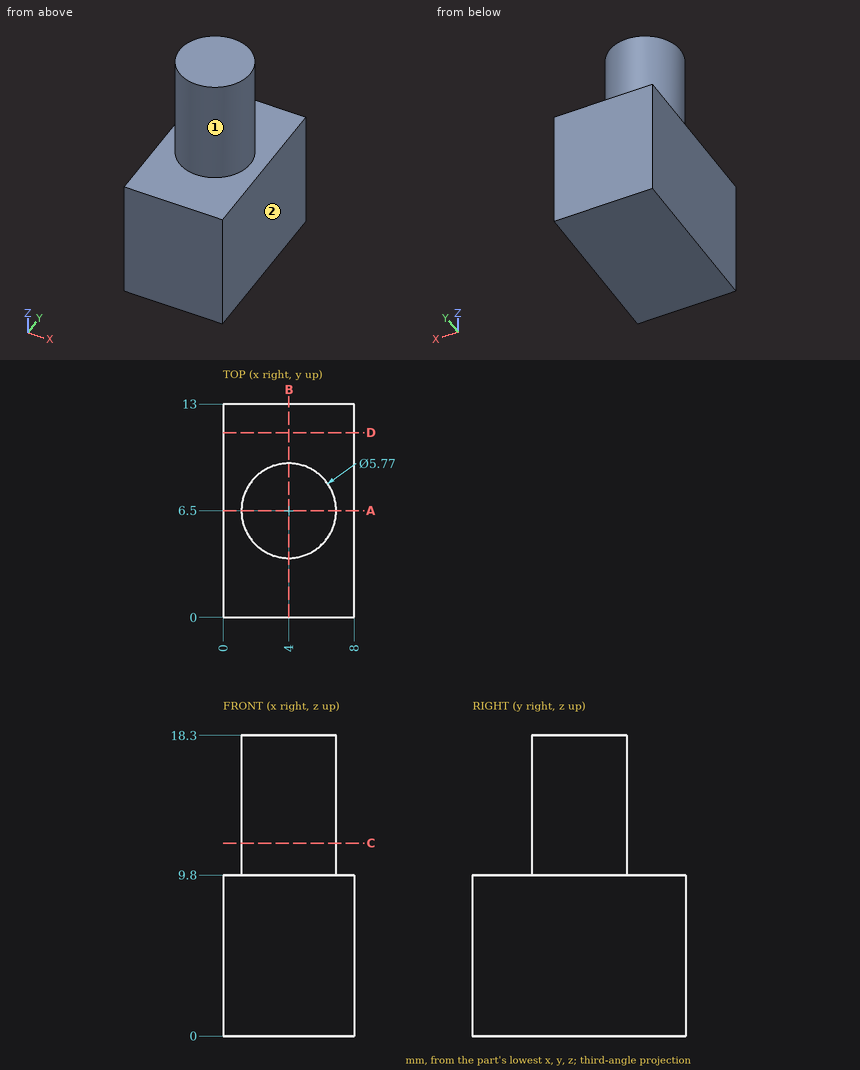
Print and shaded views of the part. All mm, measured from the part's lowest x, y and z. A direction names the side the tool comes from. Give positions to 0.01 mm unless a question says otherwise; leave off trailing zeros. Loops run counter-clockwise (first coordinate to the right, second up) from the corner with the lowest first, then second, coordinate; pieces in that order, holes last. Notation, with made-up numbers: (-31.75, -4.5) -> (25.25, -4.5) arc R22 ccw to (25.25, 11.5) -> close; hole circle Ø11 at (-18.75, 20). An arc over 180 degrees is marked (long way). Answer in a Markdown table with one row per item.
Item 1: Slice it at D-D on y = 11.25. Write the cut outline in (x, z), plus the area to 3 significant figures.
Findings below:
| item | result |
|---|---|
| outline | (0, 0) -> (8, 0) -> (8, 9.8) -> (0, 9.8) -> close |
| area | 78.4 mm² |
Item 2: Slice it at A-A on y = 6.5. Write the cut outline in (x, z) (3 decimals), plus the area to 3 significant figures.
Findings below:
| item | result |
|---|---|
| outline | (0, 0) -> (8, 0) -> (8, 9.8) -> (6.885, 9.8) -> (6.885, 18.3) -> (1.115, 18.3) -> (1.115, 9.8) -> (0, 9.8) -> close |
| area | 127 mm² |
Item 3: Tool access for the marked faces 1 and 2: list every direction of +Z, -Z, +X, -X, +Y, -Y with a clear straight run to the whole face (end or side of a thin tool).
Findings below:
| item | result |
|---|---|
| face 1 | +Z |
| face 2 | +Z, -Z, +X, +Y, -Y |
Item 4: Flat gauge pins, fed straight in: P1, Ø3, axis at y = 9, z = 5.5, coming from the -X side; P2, Ø3, axis at x = 2, z = 15.5, coming from the -Y side; P3, Ø1, axis at x = 5.5, z = 14.5, coming from the -Y side. Where does each tip first touch, or does it go through?
Findings below:
| item | result |
|---|---|
| P1 | stops at x = 0 |
| P2 | stops at y = 3.66 |
| P3 | stops at y = 3.79 |
Item 5: Slice it at B-B on x = 4. Write the cut outline in (y, z) (3 decimals), plus the area to 3 significant figures.
Findings below:
| item | result |
|---|---|
| outline | (0, 0) -> (13, 0) -> (13, 9.8) -> (9.385, 9.8) -> (9.385, 18.3) -> (3.615, 18.3) -> (3.615, 9.8) -> (0, 9.8) -> close |
| area | 176 mm² |
Item 6: Slice it at C-C on z = 11.75. Write the cut outline in (x, y) (3 decimals).
Findings below:
| item | result |
|---|---|
| outline | circle Ø5.77 at (4, 6.5) |
Item 7: Probe line 1 along Z through (x, y) = (1.25, 10); line 2 along Y through (x, z) = (3.25, 11.25); line 3 along Y through (x, z) = (5, 17). List the from-to ranges inside material, lowest first. Write a range as [from, to].
Findings below:
| item | result |
|---|---|
| line 1 | z = [0, 9.8] |
| line 2 | y = [3.71, 9.29] |
| line 3 | y = [3.79, 9.21] |
